Could you check a few things on this model? Use its own coordinates, in mm. A direction names the side the tool comes from. Coordinates: 2 decimals unless noted, no trailing zeros. Loops run counter-clockwise (first coordinate to the right, second up) from the corner with the lowest first, then second, coordinate; pieces in that order, holes last. Notation, with made-up numbers: (82, 80.25) - (96, 80.25) arc R8 cw to (96, 91.25) - close; hole circle Ø9 at (13, 59.5). An arc over 180 degrees is marked (long way). Use CSV: the item, a comma, the result in double quotes.
from build123d import *

# Parameters (mm, degrees)
SKETCH_3_R          = 8
CUT_EXTRUDE_1_DEPTH = 37


with BuildPart() as part:
    # Эскиз2 → Повернуть1 (revolve)
    with BuildSketch(Plane.XY, mode=Mode.PRIVATE) as revolve_1_sk:
        Polygon((13.5, 5.5), (14, 5.5), (14, 0), (0, 0), (0, 37), (14, 37), (14, 31.5), (13.5, 31.5), (13.5, 29.9), (14, 29.9), (14, 7.1), (13.5, 7.1), align=None)
    revolve(revolve_1_sk.sketch.rotate(Axis((0, 0, 0), (0, 1, 0)), 90), axis=Axis((0, 0, 0), (0, 1, 0)))

    # Эскиз3 → Вырез-Вытянуть1 (cut)
    with BuildSketch(Plane(origin=(0, 37, 0), x_dir=(1, 0, 0), z_dir=(0, 1, 0))):
        with Locations(Location((0, 0, 0), (0, 0, 270))):
            Circle(SKETCH_3_R)
    extrude(amount=-CUT_EXTRUDE_1_DEPTH, mode=Mode.SUBTRACT)


solid = part.part
(1) Please list where these lines run through material, in increasing order: line 1 (X direction, y = 28, z = 0); line 2 (Z direction, x = -1.75, y = 9.5); line 3 (X direction, y = 34, z = 5.25).
Computed:
line 1,"x = -14 to -8, 8 to 14"
line 2,"z = -13.89 to -7.81, 7.81 to 13.89"
line 3,"x = -12.98 to -6.04, 6.04 to 12.98"
(2) Suppose I cut it at B-B (z = 0). Write out the boundary of the cut face in (x, y), plus the area to 3 significant figures.
Computed:
outline,"(-14, 0) - (-8, 0) - (-8, 37) - (-14, 37) - (-14, 31.5) - (-13.5, 31.5) - (-13.5, 29.9) - (-14, 29.9) - (-14, 7.1) - (-13.5, 7.1) - (-13.5, 5.5) - (-14, 5.5) - close; (8, 0) - (14, 0) - (14, 5.5) - (13.5, 5.5) - (13.5, 7.1) - (14, 7.1) - (14, 29.9) - (13.5, 29.9) - (13.5, 31.5) - (14, 31.5) - (14, 37) - (8, 37) - close"
area,"441 mm²"
(3) Will these pins go through, and if not, where does the flat tip stop? pin 1 (1 mm diameter, centred on y = 11.5, z = 6, fed in from -X); pin 2 (1.5 mm diameter, centred on x = -9.5, y = 7.5, fed in from +Z); pin 3 (1.5 mm diameter, centred on y = 9.5, z = 2.5, fed in from -X).
Computed:
pin 1,"stops at x = -12.87"
pin 2,"stops at z = 10.93"
pin 3,"stops at x = -13.89"
(4) Which directions (+Z, -Z, +X, -X, +Y, -Y) give clear straight access to the entire face, cutting with the end or side of a thin tool? Please do faces 4 (the face through (12.4, 18.3, -6.5)), 5 (the face through (13.18, 6.29, 2.93)).
Computed:
face 4,"+Y, -Y"
face 5,"none"
(5) Suppose I cut it at D-D (y = 31). Write out the boundary of the cut face in (x, z).
Computed:
outline,"circle Ø27 at (0, 0); hole circle Ø16 at (0, 0)"
(6) Suppose I cut it at C-C (z = 10.5). Write out the boundary of the cut face in (x, y), plus the area to 3 significant figures.
Computed:
outline,"(-9.26, 0) - (9.26, 0) - (9.26, 5.5) - (8.49, 5.5) - (8.49, 7.1) - (9.26, 7.1) - (9.26, 29.9) - (8.49, 29.9) - (8.49, 31.5) - (9.26, 31.5) - (9.26, 37) - (-9.26, 37) - (-9.26, 31.5) - (-8.49, 31.5) - (-8.49, 29.9) - (-9.26, 29.9) - (-9.26, 7.1) - (-8.49, 7.1) - (-8.49, 5.5) - (-9.26, 5.5) - close"
area,"680 mm²"
(7) Suppose I cut it at A-A (x = 0). Write out the boundary of the cut face in (y, z).
Computed:
outline,"(0, -14) - (5.5, -14) - (5.5, -13.5) - (7.1, -13.5) - (7.1, -14) - (29.9, -14) - (29.9, -13.5) - (31.5, -13.5) - (31.5, -14) - (37, -14) - (37, -8) - (0, -8) - close; (0, 8) - (37, 8) - (37, 14) - (31.5, 14) - (31.5, 13.5) - (29.9, 13.5) - (29.9, 14) - (7.1, 14) - (7.1, 13.5) - (5.5, 13.5) - (5.5, 14) - (0, 14) - close"
(8) Thinking about a two-plate mould opening in X: for faces 1 (the face through (-7.81, 18.76, -1.73)), 2 (the face through (6, 0, -6)), 3 (the face through (13.18, 30.69, 2.93)), which applies, +X half, -X half, draft (parallel to the pull), parting line (faces both ways), or undercut?
Computed:
face 1,"undercut"
face 2,"draft"
face 3,"parting line"
